from build123d import *

# Parameters (mm, degrees)
PAD_DEPTH            = 75
SKETCH001_R          = 7.377572
PAD001_DEPTH         = 16
CHAMFER_SIZE         = 1
POCKET_DEPTH         = 13.001
POCKET_DEPTH_BACK    = -13.001
SKETCH003_R          = 4.728662
POCKET001_DEPTH      = 5
POCKET002_DEPTH      = 0.001
POCKET002_DEPTH_BACK = -27.579089
SKETCH005_R          = 1.899906
POCKET003_DEPTH      = 5


with BuildPart() as part:
    # Sketch → Pad (new body)
    with BuildSketch(Plane.XY):
        with BuildLine():
            ThreePointArc((-11.354577, 11.354577), (-13, 0), (-11.354577, -11.354577))
            ThreePointArc((-11.354577, -11.354577), (0, -13), (11.354577, -11.354577))
            ThreePointArc((11.354577, -11.354577), (13, 0), (11.354577, 11.354577))
            ThreePointArc((11.354577, 11.354577), (0, 13), (-11.354577, 11.354577))
        make_face()
    extrude(amount=PAD_DEPTH)

    # Sketch001 (on Face6 of Pad) → Pad001 (join)
    with BuildSketch(Plane.XY.offset(75)):
        Circle(SKETCH001_R)
    extrude(amount=PAD001_DEPTH)

    # Chamfer
    chamfer_edges = [part.edges().sort_by_distance(p)[0] for p in [
        (-7.377572, 0, 91),
    ]]
    chamfer(chamfer_edges, length=CHAMFER_SIZE)

    # Sketch002 → Pocket (cut, two sides)
    with BuildSketch(Plane.YZ) as pocket_sk:
        Polygon((0, 0), (-18.582906, 23.128181), (-18.582906, -17.102173), (18.582906, -17.102173), (18.582906, 23.128181), align=None)
    extrude(amount=-POCKET_DEPTH, mode=Mode.SUBTRACT)
    extrude(pocket_sk.sketch, amount=-POCKET_DEPTH_BACK, mode=Mode.SUBTRACT)

    # Sketch003 (on DatumPlane) → Pocket001 (cut)
    with BuildSketch(Plane(origin=(0, 13.444963, 45.243954), x_dir=(1, 0, 0), z_dir=(0, 1, -0.000512))):
        with Locations((0, 20.195527)):
            Circle(SKETCH003_R)
    extrude(amount=-POCKET001_DEPTH, mode=Mode.SUBTRACT)

    # Sketch004 (on DatumPlane) → Pocket002 (cut, two sides)
    with BuildSketch(Plane(origin=(-14.478585, 0, 40.939498), x_dir=(0, 1, 0), z_dir=(0.999997, 0, -0.002433))) as pocket002_sk:
        with BuildLine():
            ThreePointArc((-4.143615, -19.031831), (0, -23.175446), (4.143615, -19.031831))
            Line((4.143615, -19.031831), (4.143615, 15.684834))
            Line((-15.203477, 30.408852), (4.143615, 15.684834))
            Line((-15.203477, 30.408852), (-20.945486, 20.160222))
            Line((-4.143615, 7.373234), (-20.945486, 20.160222))
            Line((-4.143615, -19.031831), (-4.143615, 7.373234))
        make_face()
    extrude(amount=-POCKET002_DEPTH, mode=Mode.SUBTRACT)
    extrude(pocket002_sk.sketch, amount=-POCKET002_DEPTH_BACK, mode=Mode.SUBTRACT)

    # Sketch005 (on Face18 of Pocket002) → Pocket003 (cut)
    with BuildSketch(Plane(origin=(0, 8.421799, -0.004311), x_dir=(-1, 0, 0), z_dir=(0, 1, -0.000512))):
        with Locations((0, 25.085957)):
            Circle(SKETCH005_R)
    extrude(amount=-POCKET003_DEPTH, mode=Mode.SUBTRACT)


solid = part.part
Model file for the job. Use its own axes, mm. A direction names the side the tool comes from. Coordinates: 2 decimals unless noted, no trailing zeros. Write each loop counter-clockwise with the first axis right and the second up, starting at its lowest first coordinate (ties: lowest second). Pieces come first, ordered by that corner, then holes. Notation, with made-up numbers: (-3.5, -15) - (35.5, -15) arc R14 cw to (35.5, 2) - close; hole circle Ø11 at (26.25, -32). An arc over 180 degrees is marked (long way). Write each question's results on one line, items separated by ' | '. Start each with the question number.
1) Probe line 1 along Y through (x, z) = (-7.75, 33); line 2 along Z through (x, y) = (-4, 11.25); line 3 along Z through (x, y) = (-5.5, -7.75). List the from-to ranges inside material, lowest first. Write a range as from..to.
2) 3-axis set-ups, long thin cutter, end or side, ignore diameter. For faces 1 (the face through (-6, -6, 75)), 2 (the face through (0, -4.144, 35)): which of +Z, -Z, +X, -X, +Y, -Y reach the whole face in a straight line?
3) Cut at C-C (z = 84.5). Write the cut outline in (x, y).
4) Cut at A-A (z = 44). Write the cut outline in (x, y), then the cut area to 3 significant figures.
5) Mould opens along X. For faces 3 (the face through (-4.724, 10.75, 24.842)), 4 (the face through (12.7, 4.9, 37)), 5 (the face through (0, 13, 44)), 6 (the face through (0, 0, 91)) say: pulls with the +X half, pulls with the -X half, needs draft (parallel to the pull), parting line crosses it, or undercut.
6) Cut at B-B (y = -9.25). Write the cut outline in (x, z).
7) Flat gauge pins, fed straight in: P1, Ø1, axis at x = -4.5, y = -2, coming from the -Z side; P2, Ø8, axis at y = -1.5, z = 34.5, coming from the +X side; P3, Ø4, axis at x = 3.5, y = 7, coming from the -Z side. Where does each tip first touch, or does it go through?
Returned:
1) line 1: -12.24..-4.14, 4.14..12.24 | line 2: 14..22.53, 27.57..75 | line 3: 9.65..51.04, 65.65..75
2) face 1: +Z | face 2: +X, -X
3) outline: circle Ø14.76 at (0, 0)
4) outline: (-12.78, -4.14) arc R40 ccw to (-11.35, -11.35) arc R40 ccw to (11.35, -11.35) arc R40 ccw to (12.78, -4.14) - close; (-12.78, 4.14) - (12.78, 4.14) arc R40 ccw to (11.35, 11.35) arc R40 ccw to (-11.35, 11.35) arc R40 ccw to start | area: 401 mm^2
5) face 3: undercut | face 4: pulls with the +X half | face 5: parting line crosses it | face 6: needs draft
6) outline: (-11.92, 11.51) - (11.92, 11.51) - (11.92, 52.13) - (-11.92, 52.19) - close; (-11.92, 66.81) - (11.92, 66.75) - (11.92, 75) - (-11.92, 75) - close
7) P1: z = 1.87 | P2: x = 12.78 | P3: z = 6.22
